Design review of the part built by this model. Coordinates are the model's own, in mm. Coordinates: 2 decimals unless noted, no trailing zeros. Write each loop counter-clockwise with the first axis right and the second up, starting at its lowest first coordinate (ties: lowest second). Pieces come first, ordered by that corner, then holes. Notation, with made-up numbers: (65.5, 67.25) -> (79.5, 67.25) arc R26 ccw to (79.5, 104.25) -> close; hole circle Ø10 at (-26, 27). An arc over 180 degrees is marked (long way). Write item = value, one per line. Start each with the question number.
```python
from build123d import *

# Parameters (mm, degrees)
IZIM2_R               = 0.5
KES_EKSTR_ZYON1_DEPTH = 10
IZIM4_W               = 23.900856007
IZIM4_H               = 1
IZIM4_W_2             = 0.459530198
KES_EKSTR_ZYON2_DEPTH = 10
KES_EKSTR_ZYON3_DEPTH = 0.3
IZIM6_R               = 0.5
KES_EKSTR_ZYON4_DEPTH = 7
IZIM7_R               = 0.5
KES_EKSTR_ZYON5_DEPTH = 5


with BuildPart() as part:
    # Süpür1: sweep along a path in Çizim1
    with BuildLine(Plane.XY) as s_p_r1_path:
        Line((0, 0), (50.361666029, 0))
    # Çizim2 → Süpür1 (sweep)
    with BuildSketch(Plane(origin=(50.361666029, 0, 0), x_dir=(0, 0, -1), z_dir=(1, 0, 0))):
        Circle(IZIM2_R)
    sweep(path=s_p_r1_path.line)

    # Çizim3 → Kes-Ekstrüzyon1 (cut)
    with BuildSketch(Plane.XY):
        Polygon((25.974112066, 2.781879013), (25.974112066, -2.743425523), (51.839823407, -2.743425523), (51.839823407, 3.328337703), align=None)
    extrude(amount=-KES_EKSTR_ZYON1_DEPTH, mode=Mode.SUBTRACT)

    # Çizim4 → Kes-Ekstrüzyon2 (cut)
    with BuildSketch(Plane(origin=(0, 0, 0), x_dir=(-1, 0, 0), z_dir=(0, 0, -1))):
        with Locations((-38.411238026, 0)):
            Rectangle(IZIM4_W, IZIM4_H)
        with Locations((-26.203877165, 0)):
            Rectangle(IZIM4_W_2, IZIM4_H)
    extrude(amount=-KES_EKSTR_ZYON2_DEPTH, mode=Mode.SUBTRACT)


with BuildPart() as kes_ekstr_zyon2_piece_1:
    # of the separate pieces the step leaves, piece 1, a body of its own (kes_ekstr_zyon2_pieces)
    add(part.part.solids().sort_by_distance((0, 0, -0.5))[0])

    # Çizim6 → Kes-Ekstrüzyon4 (cut)
    with BuildSketch(Plane(origin=(0, 0, 0), x_dir=(0, 0, -1), z_dir=(1, 0, 0))):
        Circle(IZIM6_R)
    extrude(amount=KES_EKSTR_ZYON4_DEPTH, mode=Mode.SUBTRACT)

    # Çizim7 → Kes-Ekstrüzyon5 (cut)
    with BuildSketch(Plane.ZY.offset(-7)):
        Circle(IZIM7_R)
    extrude(amount=-KES_EKSTR_ZYON5_DEPTH, mode=Mode.SUBTRACT)


with BuildPart() as kes_ekstr_zyon2_piece_2:
    # of the separate pieces the step leaves, piece 2, a body of its own (kes_ekstr_zyon2_pieces)
    add(part.part.solids().sort_by_distance((26.433642264, 0.5, 0))[0])

    # Çizim5 → Kes-Ekstrüzyon3 (cut)
    with BuildSketch(Plane(origin=(26.460810022, 0, 0), x_dir=(0, 0, -1), z_dir=(1, 0, 0))):
        with BuildLine():
            Line((0, 0.5), (0, -0.5))
            ThreePointArc((0, -0.5), (-0.5, 0), (0, 0.5))
        make_face()
    extrude(amount=-KES_EKSTR_ZYON3_DEPTH, mode=Mode.SUBTRACT)


solid = kes_ekstr_zyon2_piece_1.part
```
(1) Take a section at B-B, the plane z = -0.3. State the section outline as (x, y) points.
(2) For line 1 (Z direction, x = 25, y = 0.05); line 2 (Z direction, x = 13.5, y = -0.4), list the stretches that pass through material, from the lowest coordinate up.
(3) Take a section at A-A, the plane x = 16.5. State the section outline as (y, z) points.
(4) Take a section at C-C, the plane y = -0.25. State the section outline as (x, z) points.
Report:
q1.outline = (12, -0.4) -> (25.97, -0.4) -> (25.97, 0.4) -> (12, 0.4) -> close
q2.line_1 = -0.5 to 0.5
q2.line_2 = -0.3 to 0.3
q3.outline = circle Ø1 at (0, 0)
q4.outline = (12, -0.43) -> (25.97, -0.43) -> (25.97, 0.43) -> (12, 0.43) -> close
